```python
from build123d import *

# Parameters (mm, degrees)
BOSS_EXTRUDE1_DEPTH = 3
SKETCH2_R           = 1.5
CUT_EXTRUDE1_DEPTH  = 3


with BuildPart() as part:
    # Sketch1 → Boss-Extrude1 (new body)
    with BuildSketch(Plane.XY):
        with BuildLine():
            Line((-52.51020312, -2.31327399), (47.128491464, 3.68672601))
            ThreePointArc((47.128491464, 3.68672601), (64.120955569, -12.31327399), (47.128491464, -28.31327399))
            Line((47.128491464, -28.31327399), (-52.51020312, -22.31327399))
            ThreePointArc((-52.51020312, -22.31327399), (-61.926141798, -12.31327399), (-52.51020312, -2.31327399))
        make_face()
    extrude(amount=BOSS_EXTRUDE1_DEPTH)

    # Sketch2 → Cut-Extrude1 (cut)
    with BuildSketch(Plane.XY.offset(3)):
        with Locations((12.091972574, -12.31327399)):
            Circle(SKETCH2_R)
        with Locations((-15.908027426, -12.31327399)):
            Circle(SKETCH2_R)
        with Locations((-51.908027426, -12.31327399)):
            Circle(SKETCH2_R)
        with BuildLine():
            Line((18.75680016, -8.728910804), (47.50542085, -6.040638414))
            ThreePointArc((47.50542085, -6.040638414), (54.391972574, -12.31327399), (47.50542085, -18.585909567))
            Line((47.50542085, -18.585909567), (18.75680016, -15.897637177))
            ThreePointArc((18.75680016, -15.897637177), (15.491972574, -12.31327399), (18.75680016, -8.728910804))
        make_face()
    extrude(amount=-CUT_EXTRUDE1_DEPTH, mode=Mode.SUBTRACT)


solid = part.part
```
For this review, take the finished solid that the model builds, in its own axes (mm). A direction names the side the tool comes from. Coordinates: 2 decimals unless noted, no trailing zeros. Write each loop counter-clockwise with the first axis right and the second up, starting at its lowest first coordinate (ties: lowest second). Pieces come first, ordered by that corner, then holes. Notation, with made-up numbers: (86.25, 73) - (130.25, 73) arc R17 ccw to (130.25, 78) - close; hole circle Ø3 at (-23.5, 31). An arc over 180 degrees is marked (long way). Answer in a Markdown table with one row per item. Add a question column.
Q1. For probe 1 along Y at (x, z) = (25.5, 2.2); probe 2 along Y at (x, z) = (28, 1.95); probe 3 along Y at (x, z) = (-41, 1.55), list the stretches that pass through material, from the lowest coordinate up.
Q2. We need section B-B, the plane y = -17.5. State the section outline as (x, z) points.
Q3. We need section C-C, the plane z = 1.7. State the section outline as (x, y) points.
Q4. We need section A-A, the plane x = 24.5. State the section outline as (y, z) points.
Q5. Tool access review of faces 4 (the flat face through (32.93, -7.404, 1.521)), 5 (the cylindrical face through (-61.924, -12.525, 1.479)): name each direction out of +Z, -Z, +X, -X, +Y, -Y from which nothing blocks a thin tool from reaching the whole face with its end or side.
Q6. Draft analysis for pull direction X (two halves, no side actions). For faces 1 (the flat face through (2, -12, 0)), 2 (the flat face through (-3.388, 0.645, 1.479)), 3 (the flat face through (33.33, -17.26, 1.52)), state which applies: +X half, -X half, draft (parallel to the pull), parting line (faces both ways), or undercut.
Q7. For P1, Ø10, axis at x = -37.5, y = -22, coming from the -Z side; P2, Ø11.5, axis at x = 48.09, y = -12.31, coming from the +Z side, all flat-tipped, find the tip position at first contact; note any pin that passes through.
Q8. We need section D-D, the plane x = -44. State the section outline as (y, z) points, and give its area (3 significant figures).
Answer list:
| question | item | result |
|---|---|---|
| 1 | probe 1 | y = -27.01 to -16.53, -8.1 to 2.38 |
| 1 | probe 2 | y = -27.16 to -16.76, -7.86 to 2.53 |
| 1 | probe 3 | y = -23.01 to -1.62 |
| 2 | outline | (-60.48, 0) - (35.89, 0) - (35.89, 3) - (-60.48, 3) - close; (51.67, 0) - (63.26, 0) - (63.26, 3) - (51.67, 3) - close |
| 3 | outline | (-52.51, -22.31) - (47.13, -28.31) arc R16.03 ccw (long way) to (47.13, 3.69) - (-52.51, -2.31) arc R10.02 ccw to start; hole circle Ø3 at (-51.91, -12.31); hole circle Ø3 at (-15.91, -12.31); hole circle Ø3 at (12.09, -12.31); hole (18.76, -15.9) - (47.51, -18.59) arc R6.3 ccw (long way) to (47.51, -6.04) - (18.76, -8.73) arc R3.6 ccw to start |
| 4 | outline | (-26.95, 0) - (-16.43, 0) - (-16.43, 3) - (-26.95, 3) - close; (-8.19, 0) - (2.32, 0) - (2.32, 3) - (-8.19, 3) - close |
| 5 | face 4 | +Z, -Z |
| 5 | face 5 | +Z, -Z, -X |
| 6 | face 1 | draft |
| 6 | face 2 | -X half |
| 6 | face 3 | undercut |
| 7 | P1 | stops at z = 0 |
| 7 | P2 | passes through |
| 8 | outline | (-22.83, 0) - (-1.8, 0) - (-1.8, 3) - (-22.83, 3) - close |
| 8 | area | 63.1 mm2 |
